For this review, take the finished solid that the model builds, in its own axes (mm). A direction names the side the tool comes from. Give positions to 0.01 mm unless a question says otherwise; leave off trailing zeros. Order: outer loops, then holes, each group sorted by start corner. A loop starts at its lowest first (then second) coordinate and runs counter-clockwise, first axis right, second up. Notation, with made-up numbers: (46, 76.25) - (56, 76.25) arc R17 ccw to (56, 97.25) - close; hole circle Ø5 at (-14, 33). An arc over 180 degrees is marked (long way). Use a Markdown table: item, result. Add a question column.
1) Machinability: for faces 1 (the face through (13, 20, 4)), 2 (the face through (-64.8, 13, -0.3)), 3 (the face through (-64, 11.48, 19.21)), 4 (the face through (-39, 10, -15)), which of the approach directions +Z, -Z, +X, -X, +Y, -Y give a long, thin tool a straight path to every point of the face, cutting with its end or side? Answer none if there is none.
2) Mouldability with a two-part tool opening along X and no side actions: class faces 5 (the face through (-42, 0, 0)), 6 (the face through (-39.44, 4.93, -22.465)), 7 (the face through (-13.74, 19.72, 0.49)) as released by +X, released by -X, zero draft, split by the parting line, or undercut.
3) We need section D-D on y = 37. Write out the cut boundary in (x, z).
4) We need section A-A on z = 0. Write out the cut boundary in (x, y), then the cut area to 3 significant figures.
5) We need section B-B on y = 11. Write out the cut boundary in (x, z), then the cut area to 3 significant figures.
6) Clearance check with flat-ended pins moving along their axes: P1, Ø15, axis at x = -61, z = -3.5, coming from the +Y side; P2, Ø4.5, axis at x = 13.5, y = 21.5, coming from the +Z side; P3, Ø5, axis at y = 12, z = -5.5, coming from the +X side. State where each tip first meets the part, or that it passes through.
7) Wall thickness on L1, parallel to X at y = 11.5, z = 0; L2, parallel to Z at x = -1.25, y = 19.5; L3, parallel to X at y = 14, z = 0: over which ranges is each line inside the solid? List them lowest first.
```python
from build123d import *

# Parameters (mm, degrees)
EXTRUDE_6_DEPTH         = 10
CUT_EXTRUDE_START       = -10
CUT_EXTRUDE_3_DEPTH     = 10
EXTRUDE_3_DEPTH         = 3
SKETCH_20_R             = 20.039024427
EXTRUDE_7_DEPTH         = 30
RIB_START               = -5
RIB_1_DEPTH             = 10
HOLE_WIZARD_25_0_25_1_D = 25
SKETCH_24_W             = 14.5
SKETCH_24_H             = 8
CUT_EXTRUDE_4_DEPTH     = 93.870878105


# Read off the part's stored shape, not the designer's step: 切除-拉伸3, 筋1
with BuildPart() as part:
    # 草图17 → 凸台-拉伸6 (new body)
    with BuildSketch(Plane(origin=(0, 0, 0), x_dir=(1, 0, 0), z_dir=(0, 1, 0))):
        with BuildLine():
            Line((-80, 25), (-80, -25))
            Line((-80, -25), (0, -20))
            ThreePointArc((0, -20), (18.789024427, 0), (0, 20))
            Line((0, 20), (-80, 25))
        make_face()
    extrude(amount=EXTRUDE_6_DEPTH)

    # 切除-拉伸3 outline → 切除-拉伸3 (cut)
    with BuildSketch(Plane(origin=(0, 10, 0), x_dir=(1, 0, 0), z_dir=(0, 1, 0)).offset(CUT_EXTRUDE_START)):
        with BuildLine():
            ThreePointArc((-80, -15), (-65, 0), (-80, 15))
            Line((-80, 15), (-80, -15))
        make_face()
    extrude(amount=CUT_EXTRUDE_3_DEPTH, mode=Mode.SUBTRACT)

    # 草图19 → 拉伸-薄壁3 (add)
    with BuildSketch(Plane(origin=(0, 10, 0), x_dir=(1, 0, 0), z_dir=(0, 1, 0))):
        with BuildLine():
            ThreePointArc((-80, 25), (-55, 0), (-80, -25))
            Line((-80, -25), (-80, -15))
            ThreePointArc((-80, -15), (-65, 0), (-80, 15))
            Line((-80, 15), (-80, 25))
        make_face()
    extrude(amount=EXTRUDE_3_DEPTH)

    # 草图20 → 凸台-拉伸7 (add)
    with BuildSketch(Plane(origin=(0, 10, 0), x_dir=(1, 0, 0), z_dir=(0, 1, 0))):
        with Locations(Location((-1.25, 0, 0), (0, 0, 86.423665625))):
            Circle(SKETCH_20_R)
    extrude(amount=EXTRUDE_7_DEPTH)

    # 筋1 outline → 筋1 (add)
    with BuildSketch(Plane.XY.offset(RIB_START)):
        Polygon((-20.65521837, 32.930470155), (-50, 13), (-57, 13), (-57, 10), (-19, 10), (-19, 34), (-19.080487844, 34), align=None)
    extrude(amount=RIB_1_DEPTH)

    # Ø25.0 (25) 直径孔1 (through all)
    with Locations(Plane(origin=(0, 40, 0), x_dir=(1, 0, 0), z_dir=(0, 1, 0))):
        with Locations((-1.25, 0)):
            Hole(HOLE_WIZARD_25_0_25_1_D / 2)

    # 草图24 → 切除-拉伸4 (cut, through all)
    with BuildSketch(Plane(origin=(0, 40, 0), x_dir=(1, 0, 0), z_dir=(0, 1, 0))):
        with Locations((7.25, 0)):
            Rectangle(SKETCH_24_W, SKETCH_24_H)
    extrude(amount=-CUT_EXTRUDE_4_DEPTH, mode=Mode.SUBTRACT)


solid = part.part
```
Checked values:
| question | item | result |
|---|---|---|
| 1 | face 1 | +Y, -Y |
| 1 | face 2 | +Z, -Z, -X, +Y |
| 1 | face 3 | +Z, +Y |
| 1 | face 4 | -Z, +Y |
| 2 | face 5 | zero draft |
| 2 | face 6 | released by +X |
| 2 | face 7 | undercut |
| 3 | outline | circle Ø40.08 at (-1.25, 0); hole (10.59, -4) - (14.5, -4) - (14.5, 4) - (10.59, 4) arc R12.5 ccw (long way) to start |
| 4 | outline | (-65, 0) - (-13.75, 0) - (-13.75, 40) - (-21.29, 40) - (-21.29, 32.5) - (-50, 13) - (-65, 13) - close; (14.5, 0) - (18.79, 0) - (18.79, 40) - (14.5, 40) - close |
| 4 | area | 1,320 mm² |
| 5 | outline | (-80, -25) arc R25 ccw to (-55.51, -5) - (-20.66, -5) arc R20.04 ccw (long way) to (-20.66, 5) - (-55.51, 5) arc R25 ccw to (-80, 25) - (-80, 15) arc R15 cw to (-80, -15) - close; hole (10.59, -4) - (14.5, -4) - (14.5, 4) - (10.59, 4) arc R12.5 ccw (long way) to start |
| 5 | area | 1,710 mm² |
| 6 | P1 | y = 13 |
| 6 | P2 | z = 15.66 |
| 6 | P3 | x = 18.56 |
| 7 | L1 | -65 to -13.75, 14.5 to 18.79 |
| 7 | L2 | -20.04 to -12.5, 12.5 to 20.04 |
| 7 | L3 | -48.53 to -13.75, 14.5 to 18.79 |
